Source: CAD feature listing. Evaluate the final solid. Frame: model axes, mm. Give positions to 0.01 mm unless a question says otherwise; leave off trailing zeros. Loops run counter-clockwise (first coordinate to the right, second up) from the corner with the lowest first, then second, coordinate; pieces in that order, holes last. Notation, with made-up numbers: (-1.75, 1) -> (37.25, 1) arc R24 ccw to (37.25, 26) -> close; hole circle Ø5 at (-32.75, -3.5). An arc over 180 degrees is marked (long way). Put each result on its own line as item: value.
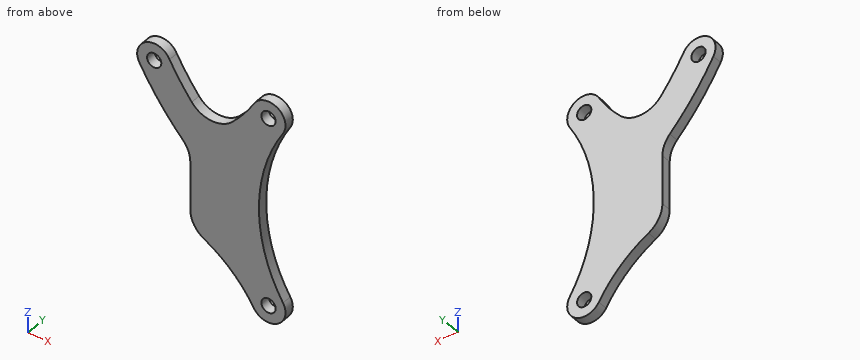
```python
from build123d import *

# Parameters (mm, degrees)
SKETCH1_R           = 2.1
BOSS_EXTRUDE1_DEPTH = 3
FILLET1_R           = 8


with BuildPart() as part:
    # Sketch1 → Boss-Extrude1 (new body)
    with BuildSketch(Plane(origin=(0, 0, 0), x_dir=(1, 0, 0), z_dir=(0, 1, 0))):
        with BuildLine():
            ThreePointArc((-6.113719472, -32.751050787), (-0.724273586, -24.461432648), (5.649824002, -16.902677739))
            ThreePointArc((5.649824002, -16.902677739), (12.975948477, -22.768180875), (18.703056171, -30.202995218))
            ThreePointArc((18.703056171, -30.202995218), (25.587038372, -31.925076677), (27.260231116, -25.029048724))
            ThreePointArc((27.260231116, -25.029048724), (20.185963894, 0), (27.260231116, 25.029048724))
            ThreePointArc((27.260231116, 25.029048724), (25.587038372, 31.925076677), (18.703056171, 30.202995218))
            ThreePointArc((18.703056171, 30.202995218), (10.659672329, 20.591511651), (0, 14))
            Line((0, 14), (0, -8.396398763))
            ThreePointArc((0, -8.396398763), (-8.177458209, -17.750627647), (-14.984135407, -28.14493216))
            ThreePointArc((-14.984135407, -28.14493216), (-12.92577576, -35.025301553), (-6.113719472, -32.751050787))
        make_face()
        with Locations(Location((-10.621571061, -30.587887812, 0), (0, 0, 270))):
            Circle(SKETCH1_R, mode=Mode.SUBTRACT)
        with Locations(Location((23, -27.646381495, 0), (0, 0, 270))):
            Circle(SKETCH1_R, mode=Mode.SUBTRACT)
        with Locations(Location((23, 27.646381495, 0), (0, 0, 270))):
            Circle(SKETCH1_R, mode=Mode.SUBTRACT)
    extrude(amount=BOSS_EXTRUDE1_DEPTH)

    # Fillet1
    fillet1_edges = [part.edges().sort_by_distance(p)[0] for p in [
        (0, 1.5, -14),
        (5.649824002, 1.5, 16.902677739),
        (0, 1.5, 8.396398763),
    ]]
    fillet(fillet1_edges, radius=FILLET1_R)


solid = part.part
```
(1) Line query: probe 1 along X at (y, z) = (0.1, 27.5); probe 2 along Z at (x, y) = (23.5, 1.35); probe 3 along X at (y, z) = (2.1, 31). Output: solid intervals per line, ascending. Write a range as from..to.
Calculated:
probe 1: x = -14.62..-2.87, 16.94..20.91, 25.09..28
probe 2: z = -32.62..-29.69, -25.61..-17.49, 17.49..25.61, 29.69..32.62
probe 3: x = -15.6..-12.68, -8.56..-5.09, 19.29..26.71
(2) Section D-D on y = 1.1. Give the number of separate pieces and of enclosed holes in the cut face, then the cut area to 3 significant figures.
Calculated:
separate pieces: 1
enclosed holes: 3
area: 1,290 mm²
(3) Section A-A on z = -27. Return loops of the section in (x, y).
Calculated:
outline: (16.58, 0) -> (21, 0) -> (21, 3) -> (16.58, 3) -> close; (25, 0) -> (27.96, 0) -> (27.96, 3) -> (25, 3) -> close
(4) First-contact query: P1, Ø1.5, axis at y = 2, z = -1, coming from the -X side; P2, Ø1, axis at x = 12.5, y = 1, coming from the -Z side. Flat tips, straight axial feed; report the tip coordinate or a pass-through.
Calculated:
P1: stops at x = 0
P2: stops at z = -22.79
(5) Section B-B on x = 23. Return loops of the section in (y, z), then the cut area to 3 significant figures.
Calculated:
outline: (0, -32.65) -> (3, -32.65) -> (3, -29.75) -> (0, -29.75) -> close; (0, -25.55) -> (3, -25.55) -> (3, -16.16) -> (0, -16.16) -> close; (0, 16.16) -> (3, 16.16) -> (3, 25.55) -> (0, 25.55) -> close; (0, 29.75) -> (3, 29.75) -> (3, 32.65) -> (0, 32.65) -> close
area: 73.7 mm²
(6) Section C-C on x = -9.5. Return loops of the section in (y, z).
Calculated:
outline: (0, 19.54) -> (3, 19.54) -> (3, 28.81) -> (0, 28.81) -> close; (0, 32.36) -> (3, 32.36) -> (3, 35.46) -> (0, 35.46) -> close
